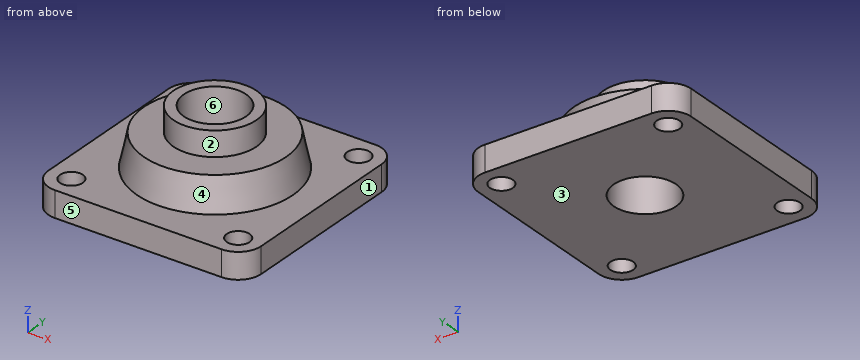
```python
from build123d import *

# Parameters (mm, degrees)
SKETCH001_R   = 7
SKETCH001_R_2 = 19.05
PAD_DEPTH     = 15.875


with BuildPart() as part:
    # Sketch → Revolution (revolve)
    with BuildSketch(Plane.XZ):
        Polygon((19.05, 0), (19.05, 51.2064), (25.4, 51.2064), (25.4, 36.068), (43.4, 36.068), (51.05, 0), align=None)
    revolve(axis=Axis((0, 0, 0), (0, 0, 1)))

    # Sketch001 → Pad (new body)
    with BuildSketch(Plane.XY):
        with BuildLine():
            ThreePointArc((-51.0032, 65.0875), (-60.962304, 60.962304), (-65.0875, 51.0032))
            Line((-65.0875, -51.0032), (-65.0875, 51.0032))
            ThreePointArc((-65.0875, -51.0032), (-60.962304, -60.962304), (-51.0032, -65.0875))
            Line((51.0032, -65.0875), (-51.0032, -65.0875))
            ThreePointArc((51.0032, -65.0875), (60.962304, -60.962304), (65.0875, -51.0032))
            Line((65.0875, 51.0032), (65.0875, -51.0032))
            ThreePointArc((65.0875, 51.0032), (60.962304, 60.962304), (51.0032, 65.0875))
            Line((-51.0032, 65.0875), (51.0032, 65.0875))
        make_face()
        with Locations((51.0032, 51.0032)):
            Circle(SKETCH001_R, mode=Mode.SUBTRACT)
        with Locations((-51.0032, 51.0032)):
            Circle(SKETCH001_R, mode=Mode.SUBTRACT)
        with Locations((-51.0032, -51.0032)):
            Circle(SKETCH001_R, mode=Mode.SUBTRACT)
        with Locations((51.0032, -51.0032)):
            Circle(SKETCH001_R, mode=Mode.SUBTRACT)
        Circle(SKETCH001_R_2, mode=Mode.SUBTRACT)
    extrude(amount=PAD_DEPTH)


solid = part.part
```
For this review, take the finished solid that the model builds, in its own axes (mm). Face numbers are marked on the shaded views. A direction names the side the tool comes from. Give positions to 0.01 mm unless a question says otherwise; leave off trailing zeros. Loops run counter-clockwise (first coordinate to the right, second up) from the corner with the lowest first, then second, coordinate; pieces in that order, holes last. Notation, with made-up numbers: M 36.25,31 L 62.25,31 A29 cw 62.25,57 Z; hole C 16,-28.75 d8. An arc over 180 degrees is marked long. One line per item, written item: value. Start each with the question number.
Q1. Add section D-D (z = 39). Give the boundary of the cut face in (x, y).
Q2. Draft analysis for pull direction Y (two halves, no side actions). For the marked faces 3, 4, 5 and 6, state which applies: released by +Y, released by -Y, zero draft, split by the parting line, or undercut.
Q3. Clearance check with flat-ended pins moving along their axes: pin 1 Ø12 at (x, y) = (22.5, -17.5) entering from +Z; pin 2 Ø8 at (x, z) = (22.5, 40.5) entering from +Y; pin 3 Ø2 at (x, z) = (-22.5, 43.5) entering from +Y; pin 4 Ø16 at (x, y) = (51, -51) entering from +Z (3 decimals). State where each tip first meets the part, or that it passes through.
Q4. Machinability: for the marked faces 1 and 2, which of the approach directions +Z, -Z, +X, -X, +Y, -Y give a long, thin tool a straight path to every point of the face, cutting with its end or side? Answer none if there is none.
Q5. Add section C-C (z = 12). Give the boundary of the cut face in (x, y), and give its area (3 significant figures).
Q6. For L1, parallel to Z at x = -57.5, y = 57 (3 decimals); L2, parallel to Z at x = -27, y = -2.5; L3, parallel to X at y = 7.5, z = 47, list the stretches that pass through material, from the lowest coordinate up.
Reply:
1. outline: C 0,0 d50.8; hole C 0,0 d38.1
2. face 3: zero draft
2. face 4: split by the parting line
2. face 5: released by -Y
2. face 6: undercut
3. pin 1: z = 51.21
3. pin 2: y = 17.4
3. pin 3: y = 13.52
3. pin 4: z = 15.875
4. face 1: +Z, -Z, +X, +Y, -Y
4. face 2: +Z
5. outline: M -65.09,-51 A14.08 ccw -51,-65.09 L 51,-65.09 A14.08 ccw 65.09,-51 L 65.09,51 A14.08 ccw 51,65.09 L -51,65.09 A14.08 ccw -65.09,51 Z; hole C -51,-51 d14; hole C -51,51 d14; hole C 0,0 d38.1; hole C 51,-51 d14; hole C 51,51 d14
5. area: 15,000 mm²
6. L1: 0 to 15.875
6. L2: 0 to 36.07
6. L3: -24.27 to -17.51, 17.51 to 24.27
